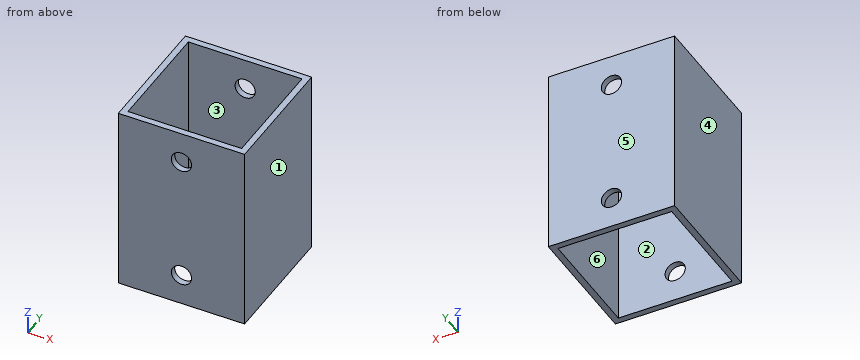
from build123d import *

# Parameters (mm, degrees)
SKETCH_1_W          = 20
SKETCH_1_H          = 20
SKETCH_1_W_2        = 18
SKETCH_1_H_2        = 18
EXTRUDE_1_DEPTH     = 30
SKETCH_2_R          = 1.6
CUT_EXTRUDE_1_DEPTH = 50


with BuildPart() as part:
    # 草图1 → 凸台-拉伸1 (new body)
    with BuildSketch(Plane.XY):
        Rectangle(SKETCH_1_W, SKETCH_1_H)
        Rectangle(SKETCH_1_W_2, SKETCH_1_H_2, mode=Mode.SUBTRACT)
    extrude(amount=EXTRUDE_1_DEPTH)

    # 草图2 → 切除-拉伸1 (cut)
    with BuildSketch(Plane(origin=(0, 10, 0), x_dir=(1, 0, 0), z_dir=(0, 1, 0))):
        with Locations(Location((0, -5, 0), (0, 0, 270))):
            Circle(SKETCH_2_R)
        with Locations(Location((0, -25, 0), (0, 0, 270))):
            Circle(SKETCH_2_R)
    extrude(amount=-CUT_EXTRUDE_1_DEPTH, mode=Mode.SUBTRACT)


solid = part.part
Build history of the part. All positions in model axes, mm. Face numbers are marked on the shaded views. A direction names the side the tool comes from. Give positions to 0.01 mm unless a question says otherwise; leave off trailing zeros. Write each loop counter-clockwise with the first axis right and the second up, starting at its lowest first coordinate (ties: lowest second). Pieces come first, ordered by that corner, then holes. Notation, with made-up numbers: (54, 47.25) - (60, 47.25) arc R13 ccw to (60, 58.25) - close; hole circle Ø6 at (-24.5, 84.25). An arc over 180 degrees is marked (long way). Use one line per item in the form item = value. Start each with the question number.
1. 3-axis set-ups, long thin cutter, end or side, ignore diameter. For the marked faces 1 and 2: which of +Z, -Z, +X, -X, +Y, -Y reach the whole face in a straight line?
2. Band-saw the part on D-D on x = 0. Write the cut outline in (y, z).
3. Band-saw the part on C-C on z = 25. Write the cut outline in (x, y).
4. Probe line 1 (Y direction, x = -8.25, z = 28.75); line 2 (X direction, y = -9.4, z = 25). List the from-to ranges inside material, lowest first. Write a range as [from, to].
5. Two-plate mould, pull along X, no slides. Class the marked faces 3, 4, 5 and 6: released by +X, released by -X, zero draft, split by the parting line, or undercut.
6. Band-saw the part on A-A on x = -3. Write the cut outline in (y, z), plus the area to 3 significant figures.
7. Drop flat-ended pins along their axis: pin 1 Ø5 at (x, z) = (0, 25) entering from -Y; pin 2 Ø2.5 at (x, z) = (0, 5) entering from +Y. Give the stop position or say it passes through.
Conclusion:
q1.face_1 = +Z, -Z, +X, +Y, -Y
q1.face_2 = +Z, -Z
q2.outline = (-10, 0) - (-9, 0) - (-9, 3.4) - (-10, 3.4) - close; (-10, 6.6) - (-9, 6.6) - (-9, 23.4) - (-10, 23.4) - close; (-10, 26.6) - (-9, 26.6) - (-9, 30) - (-10, 30) - close; (9, 0) - (10, 0) - (10, 3.4) - (9, 3.4) - close; (9, 6.6) - (10, 6.6) - (10, 23.4) - (9, 23.4) - close; (9, 26.6) - (10, 26.6) - (10, 30) - (9, 30) - close
q3.outline = (-10, -10) - (-1.6, -10) - (-1.6, -9) - (-9, -9) - (-9, 9) - (-1.6, 9) - (-1.6, 10) - (-10, 10) - close; (1.6, -10) - (10, -10) - (10, 10) - (1.6, 10) - (1.6, 9) - (9, 9) - (9, -9) - (1.6, -9) - close
q4.line_1 = [-10, -9], [9, 10]
q4.line_2 = [-10, -1.6], [1.6, 10]
q5.face_3 = undercut
q5.face_4 = released by -X
q5.face_5 = zero draft
q5.face_6 = undercut
q6.outline = (-10, 0) - (-9, 0) - (-9, 30) - (-10, 30) - close; (9, 0) - (10, 0) - (10, 30) - (9, 30) - close
q6.area = 60.0 mm²
q7.pin_1 = -10
q7.pin_2 = through
